Source: CAD feature listing. Evaluate the final solid. Frame: model axes, mm. A direction names the side the tool comes from. Round coordinates to 2 decimals unless told otherwise and drop trailing zeros. Loops run counter-clockwise (first coordinate to the right, second up) from the corner with the lowest first, then second, coordinate; pieces in that order, holes last. Notation, with made-up numbers: (49, -28.5) -> (73, -28.5) arc R14 cw to (73, -20.5) -> close; hole circle Ø5 at (72.5, 78.25). An arc over 180 degrees is marked (long way). Write item = value, one per line.
from build123d import *

# Parameters (mm, degrees)
F0_W     = 48.8410666585
F0_H     = 6
F1_DEPTH = 25
F0_H_2   = 74.675624311
F2_DEPTH = 6
F3_R     = 0.8
F4_DEPTH = 25.25


with BuildPart() as f1:
    # F0 (on Top) → F1 (new body)
    with BuildSketch(Plane.XY):
        with Locations((0, -37.3378121555)):
            Rectangle(F0_W, F0_H)
    extrude(amount=F1_DEPTH)

    # F0 (on Top) → F2 (join)
    with BuildSketch(Plane.XY):
        with Locations((0, -37.3378121555)):
            Rectangle(F0_W, F0_H)
        with Locations((0, 3)):
            Rectangle(F0_W, F0_H_2)
        with BuildLine():
            Line((4.648, 29.1621878445), (4.648, -3.6038121555))
            ThreePointArc((4.648, -3.6038121555), (0, -8.2518121555), (-4.648, -3.6038121555))
            Line((-4.648, -3.6038121555), (-4.648, 29.1621878445))
            ThreePointArc((-4.648, 29.1621878445), (0, 33.8101878445), (4.648, 29.1621878445))
        make_face(mode=Mode.SUBTRACT)
    extrude(amount=F2_DEPTH)

    # F3 (on Right) → F4 (cut, symmetric)
    with BuildSketch(Plane.YZ):
        with Locations((-34.5324325053, 5.9808787941)):
            Circle(F3_R)
    extrude(amount=F4_DEPTH, both=True, mode=Mode.SUBTRACT)


solid = f1.part
1. Set-up query: faces 4 (the face through (0, -34.338, 16)), 5 (the face through (-4.648, 13, 3)), 6 (the face through (0, 40.338, 3)). Return all of +Z, -Z, +X, -X, +Y, -Y with unobstructed straight access to the full face (end or side cutting, diameter ignored); none if empty.
Evaluation:
face_4 = +Z, +X, -X, +Y
face_5 = +Z, -Z
face_6 = +Z, -Z, +X, -X, +Y
2. Section query B-B (x = 0). Return the cut outline in (y, z), then the cut area to 3 significant figures.
Evaluation:
outline = (-40.34, 0) -> (-8.25, 0) -> (-8.25, 6) -> (-33.73, 6) arc R0.8 cw (long way) to (-34.34, 6.76) -> (-34.34, 25) -> (-40.34, 25) -> close; (33.81, 0) -> (40.34, 0) -> (40.34, 6) -> (33.81, 6) -> close
area = 344 mm²
3. Line query: probe 1 along Z at (x, y) = (-15.5, -34.5); probe 2 along X at (y, z) = (13.5, 2); probe 3 along Z at (x, y) = (10, 20.5). Output: solid intervals per line, ascending. Write a range as from..to.
Evaluation:
probe_1 = 0..5.18, 6.78..25
probe_2 = -24.42..-4.65, 4.65..24.42
probe_3 = 0..6
4. Contact query for flat-ended pins moving along their axis: pin 1 Ø1 at (x, y) = (18, 6) entering from +Z; pin 2 Ø2 at (x, z) = (-6, 15.5) entering from +Y; pin 3 Ø6 at (x, y) = (5.5, -15) entering from -Z. Output: stop coordinate, or through.
Evaluation:
pin_1 = 6
pin_2 = -34.34
pin_3 = 0
5. Section query D-D (x = -11). Return the cut outline in (y, z), then the cut area to 3 significant figures.
Evaluation:
outline = (-40.34, 0) -> (40.34, 0) -> (40.34, 6) -> (-33.73, 6) arc R0.8 cw (long way) to (-34.34, 6.76) -> (-34.34, 25) -> (-40.34, 25) -> close
area = 596 mm²
6. Section query C-C (y = 5). Return the cut outline in (x, z), then the cut area to 3 significant figures.
Evaluation:
outline = (-24.42, 0) -> (-4.65, 0) -> (-4.65, 6) -> (-24.42, 6) -> close; (4.65, 0) -> (24.42, 0) -> (24.42, 6) -> (4.65, 6) -> close
area = 237 mm²
7. Mould query, pull axis X, two halves, no side actions, for faces 1 (the face through (5, 4, 6)), 2 (the face through (4.648, 13, 3)), 3 (the face through (24.421, -6, 3)). Classes: released by +X, released by -X, zero draft, split by the parting line, or undercut.
Evaluation:
face_1 = zero draft
face_2 = undercut
face_3 = released by +X
8. Section query A-A (z = 4). Return the cut outline in (x, y).
Evaluation:
outline = (-24.42, -40.34) -> (24.42, -40.34) -> (24.42, 40.34) -> (-24.42, 40.34) -> close; hole (-4.65, -3.6) arc R4.65 ccw to (4.65, -3.6) -> (4.65, 29.16) arc R4.65 ccw to (-4.65, 29.16) -> close
